Could you check a few things on this drawing? It's one solid part, dimensions in mm from its lowest x, y, z. A direction names the side the tool comes from. Coordinates: 2 decimals unless noted, no trailing zeros. Loops run counter-clockwise (first coordinate to the right, second up) from the corner with the lowest first, then second, coordinate; pieces in that order, holes last.
1) Imagine slicing it at A-A on x = 4. Please give me the cut outline in (y, z).
2) Will these pins go through, and if not, where does the flat tip stop? P1, Ø4, axis at y = 5.5, z = 8, coming from the -X side; P2, Ø5, axis at y = 6.5, z = 3, coming from the -X side; P3, Ø2, axis at x = 16, y = 10, coming from the +Z side.
3) Imagine slicing it at C-C on z = 0.75. Please give me the cut outline in (x, y), plus the area to 3 significant figures.
4) For the marked faces 1 and 2, which set-ups out of +Z, -Z, +X, -X, +Y, -Y let a thin tool reach every point of the face, with its end or its side?
5) If I drill on line 1 along Y through (x, z) = (10, 1.4); line 2 along Z through (x, y) = (17, 12.25); line 3 along Y through (x, z) = (15.75, 1.25), over which ranges is the centre line in solid material (lowest first)?
6) Imagine slicing it at D-D on y = 10. Please give me the cut outline in (x, z), plus the area to 3 significant figures.
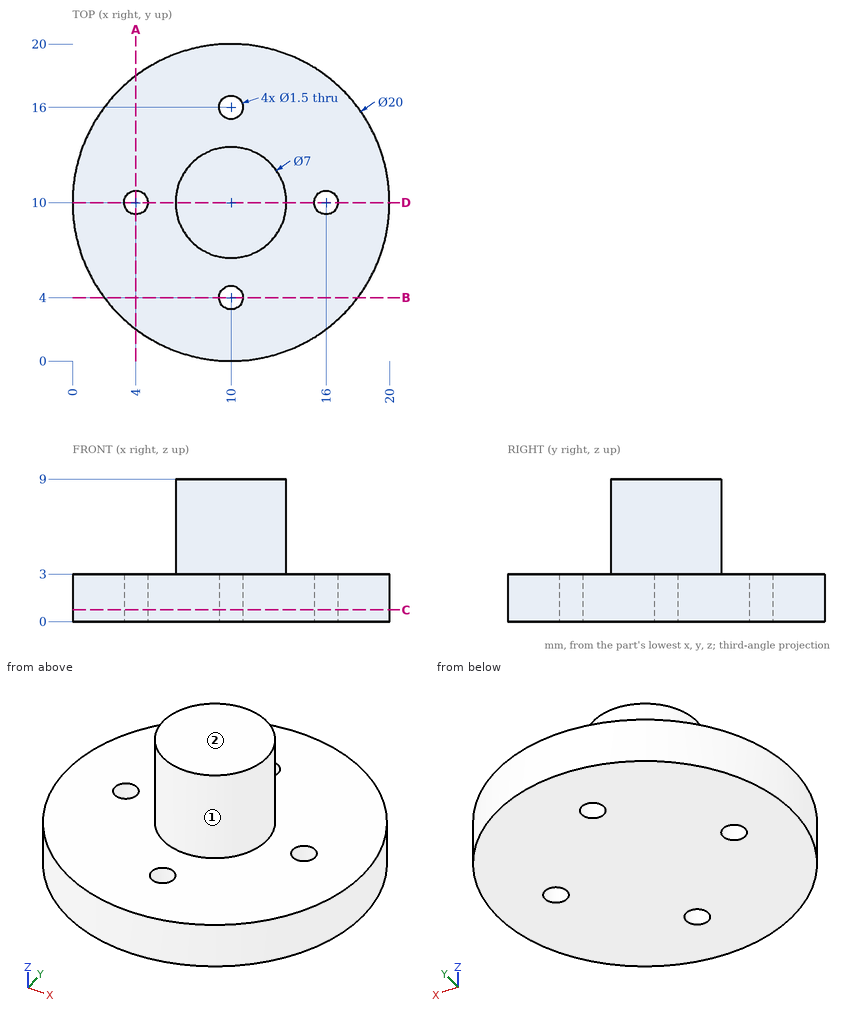
Filled in:
1. outline: (2, 0) - (9.25, 0) - (9.25, 3) - (2, 3) - close; (10.75, 0) - (18, 0) - (18, 3) - (10.75, 3) - close
2. P1: stops at x = 7.55
2. P2: stops at x = 0.05
2. P3: stops at z = 3
3. outline: circle Ø20 at (10, 10); hole circle Ø1.5 at (4, 10); hole circle Ø1.5 at (10, 4); hole circle Ø1.5 at (10, 16); hole circle Ø1.5 at (16, 10)
3. area: 307 mm2
4. face 1: +Z
4. face 2: +Z, +X, -X, +Y, -Y
5. line 1: y = 0 to 3.25, 4.75 to 15.25, 16.75 to 20
5. line 2: z = 0 to 3
5. line 3: y = 1.82 to 9.29, 10.71 to 18.18
6. outline: (0, 0) - (3.25, 0) - (3.25, 3) - (0, 3) - close; (4.75, 0) - (15.25, 0) - (15.25, 3) - (13.5, 3) - (13.5, 9) - (6.5, 9) - (6.5, 3) - (4.75, 3) - close; (16.75, 0) - (20, 0) - (20, 3) - (16.75, 3) - close
6. area: 93.0 mm2
